Source: CAD feature listing. Evaluate the final solid. Frame: model axes, mm. A direction names the side the tool comes from. Give positions to 0.01 mm unless a question says otherwise; leave off trailing zeros. Order: outer loops, then holes, each group sorted by start corner. A loop starts at its lowest first (then second) coordinate and runs counter-clockwise, first axis right, second up. Notation, with made-up numbers: (79, 17) - (114, 17) arc R35 cw to (114, 49) - close; hole circle Ø3 at (84.25, -7). An arc over 180 degrees is marked (long way). Use CSV: the item, a comma, the result in double quotes.
```python
from build123d import *

# Parameters (mm, degrees)
SKETCH1_R           = 1.75
BOSS_EXTRUDE1_DEPTH = 5
SKETCH2_R           = 1.35
BOSS_EXTRUDE2_DEPTH = 4
SKETCH4_W           = 7
SKETCH4_H           = 5
BOSS_EXTRUDE3_DEPTH = 105
BOSS_EXTRUDE4_START = -5
SKETCH5_R           = 1.75
BOSS_EXTRUDE4_DEPTH = 5
SKETCH6_R           = 1.35
CUT_EXTRUDE1_DEPTH  = 5
SKETCH8_R           = 1.5
CUT_EXTRUDE3_DEPTH  = 5


with BuildPart() as part:
    # Sketch1 → Boss-Extrude1 (new body)
    with BuildSketch(Plane.XY):
        with BuildLine():
            Line((-20.753194099, 19.75), (-20.753194099, 0))
            ThreePointArc((-20.753194099, 0), (-16.34718685, -12.785325472), (-5, -20.141873431))
            Line((-5, -20.141873431), (-5, -23.753194099))
            Line((-5, -23.753194099), (-2.5, -23.753194099))
            Line((-2.5, -23.753194099), (-2.5, -16.753194099))
            Line((-2.5, -16.753194099), (2.5, -16.753194099))
            Line((2.5, -16.753194099), (2.5, -23.753194099))
            Line((2.5, -23.753194099), (5, -23.753194099))
            Line((5, -23.753194099), (5, -20.141873431))
            ThreePointArc((5, -20.141873431), (16.34718685, -12.785325472), (20.753194099, 0))
            Line((20.753194099, 0), (20.753194099, 19.75))
            Line((20.753194099, 19.75), (13.753194099, 19.75))
            Line((13.753194099, 19.75), (13.753194099, 0))
            ThreePointArc((13.753194099, 0), (0, -13.753194099), (-13.753194099, 0))
            Line((-13.753194099, 0), (-13.753194099, 19.75))
            Line((-13.753194099, 19.75), (-20.753194099, 19.75))
        make_face()
        with Locations((-17.253194099, 10)):
            Circle(SKETCH1_R, mode=Mode.SUBTRACT)
        with Locations((-17.253194099, 0)):
            Circle(SKETCH1_R, mode=Mode.SUBTRACT)
        with Locations((17.253194099, 0)):
            Circle(SKETCH1_R, mode=Mode.SUBTRACT)
        with Locations((17.253194099, 10)):
            Circle(SKETCH1_R, mode=Mode.SUBTRACT)
    extrude(amount=BOSS_EXTRUDE1_DEPTH)

    # Sketch2 → Boss-Extrude2 (add)
    with BuildSketch(Plane(origin=(0, 0, 0), x_dir=(-1, 0, 0), z_dir=(0, 0, -1))):
        with Locations((17.253194099, 16.75)):
            Circle(SKETCH2_R)
        with Locations(Location((-17.253194099, 16.75, 0), (0, 0, 180))):
            Circle(SKETCH2_R)
    extrude(amount=BOSS_EXTRUDE2_DEPTH)

    # Sketch4 → Boss-Extrude3 (add)
    with BuildSketch(Plane(origin=(0, 0, 0), x_dir=(-1, 0, 0), z_dir=(0, 0, -1))):
        with Locations((17.253194099, 17.25)):
            Rectangle(SKETCH4_W, SKETCH4_H)
        with Locations((-17.253194099, 17.25)):
            Rectangle(SKETCH4_W, SKETCH4_H)
    extrude(amount=-BOSS_EXTRUDE3_DEPTH)

    # Sketch5 → Boss-Extrude4 (add)
    with BuildSketch(Plane.XY.offset(105).offset(BOSS_EXTRUDE4_START)):
        with BuildLine():
            Line((20.753194099, 14.75), (13.753194099, 14.75))
            Line((13.753194099, 14.75), (13.753194099, 0))
            ThreePointArc((13.753194099, 0), (0, -13.753194099), (-13.753194099, 0))
            Line((-13.753194099, 0), (-13.753194099, 14.75))
            Line((-13.753194099, 14.75), (-20.753194099, 14.75))
            Line((-20.753194099, 14.75), (-20.753194099, 0))
            ThreePointArc((-20.753194099, 0), (-16.34718685, -12.785325472), (-5, -20.141873431))
            Line((-5, -20.141873431), (-5, -23.753194099))
            Line((-5, -23.753194099), (-2.5, -23.753194099))
            Line((-2.5, -23.753194099), (-2.5, -16.753194099))
            Line((-2.5, -16.753194099), (2.5, -16.753194099))
            Line((2.5, -16.753194099), (2.5, -23.753194099))
            Line((2.5, -23.753194099), (5, -23.753194099))
            Line((5, -23.753194099), (5, -20.141873431))
            ThreePointArc((5, -20.141873431), (16.34718685, -12.785325472), (20.753194099, 0))
            Line((20.753194099, 0), (20.753194099, 14.75))
        make_face()
        with Locations((17.253194099, 10)):
            Circle(SKETCH5_R, mode=Mode.SUBTRACT)
        with Locations((-17.253194099, 10)):
            Circle(SKETCH5_R, mode=Mode.SUBTRACT)
        with Locations((-17.253194099, 0)):
            Circle(SKETCH5_R, mode=Mode.SUBTRACT)
        with Locations((17.253194099, 0)):
            Circle(SKETCH5_R, mode=Mode.SUBTRACT)
    extrude(amount=BOSS_EXTRUDE4_DEPTH)

    # Sketch6 → Cut-Extrude1 (cut)
    with BuildSketch(Plane.XY.offset(105)):
        with Locations((17.253194099, 16.75)):
            Circle(SKETCH6_R)
        with Locations(Location((-17.253194099, 16.75, 0), (0, 0, 180))):
            Circle(SKETCH6_R)
    extrude(amount=-CUT_EXTRUDE1_DEPTH, mode=Mode.SUBTRACT)

    # Sketch8 → Cut-Extrude3 (cut)
    with BuildSketch(Plane.XY.offset(105)):
        with Locations((17.253194099, 16.75)):
            Circle(SKETCH8_R)
        with Locations((-17.253194099, 16.75)):
            Circle(SKETCH8_R)
    extrude(amount=-CUT_EXTRUDE3_DEPTH, mode=Mode.SUBTRACT)


solid = part.part
```
Item 1: First-contact query: pin 1 (3.5 mm diameter, centred on x = 18.5, z = 46.5, fed in from -Y); pin 2 (3 mm diameter, centred on y = -22, z = 2, fed in from -X); pin 3 (1.5 mm diameter, centred on y = -22, z = 3, fed in from +X). Flat tips, straight axial feed; report the tip coordinate or a pass-through.
Filled in:
pin 1,"stops at y = 14.75"
pin 2,"stops at x = -5"
pin 3,"stops at x = 5"
Item 2: Section B-B on z = 67. Return the cut outline in (x, y).
Filled in:
outline,"(-20.75, 14.75) - (-13.75, 14.75) - (-13.75, 19.75) - (-20.75, 19.75) - close; (13.75, 14.75) - (20.75, 14.75) - (20.75, 19.75) - (13.75, 19.75) - close"
Item 3: Set-up query: faces 1 (the flat face through (-5, -22, 2)), 2 (the flat face through (17, 14.75, 52)), 3 (the cylindrical face through (-15.904, 16.809, -1.972)), 4 (the flat face through (2.5, -20, 2)), 5 (the flat face through (17, 17, 100)). Return all of +Z, -Z, +X, -X, +Y, -Y with unobstructed straight access to the full face (end or side cutting, diameter ignored); none if empty.
Filled in:
face 1,"+Z, -Z, -X, -Y"
face 2,"+X, -X, -Y"
face 3,"-Z"
face 4,"+Z, -Z, -Y"
face 5,"+Z"
Item 4: Mould query, pull axis Y, two halves, no side actions, for faces 6 (the cylindrical face through (0.3, -13.75, 102.46)), 7 (the flat face through (-2.5, -20, 2)), 8 (the cylindrical face through (15.96, 11.18, 2.46)). Classes: released by +Y, released by -Y, zero draft, split by the parting line, or undercut.
Filled in:
face 6,"released by +Y"
face 7,"zero draft"
face 8,"undercut"
Item 5: Section C-C on y = 10. Count the separate pieces of the cut face and the enclosed holes in it, then the cut area to 3 significant figures.
Filled in:
separate pieces,"8"
enclosed holes,"0"
area,"70.0 mm2"
Item 6: Section A-A on y = 16.75. Return the cut outline in (x, z).
Filled in:
outline,"(-20.75, 0) - (-18.6, 0) - (-18.6, -4) - (-15.9, -4) - (-15.9, 0) - (-13.75, 0) - (-13.75, 105) - (-15.75, 105) - (-15.75, 100) - (-18.75, 100) - (-18.75, 105) - (-20.75, 105) - close; (13.75, 0) - (15.9, 0) - (15.9, -4) - (18.6, -4) - (18.6, 0) - (20.75, 0) - (20.75, 105) - (18.75, 105) - (18.75, 100) - (15.75, 100) - (15.75, 105) - (13.75, 105) - close"
Item 7: Material intervals for line 1 (Z direction, x = -17, y = 5.5); line 2 (X direction, y = 18.5, z = 10.5); line 3 (X direction, y = 16, z = 102), sorted ascending. Write a range as from..to.
Filled in:
line 1,"z = 0..5, 100..105"
line 2,"x = -20.75..-13.75, 13.75..20.75"
line 3,"x = -20.75..-18.55, -15.95..-13.75, 13.75..15.95, 18.55..20.75"
